```python
from build123d import *

# Parameters (mm, degrees)
F0_W     = 27
F0_H     = 31
F1_DEPTH = 2.5
F2_W     = 20.5
F2_H     = 31
F3_DEPTH = 2.5
F4_W     = 20.5
F4_H     = 31
F5_DEPTH = 2.5
F6_R     = 1.5
F7_DEPTH = 20.501
F8_R     = 1.5
F9_DEPTH = 32.001


with BuildPart() as f1:
    # F0 (on Right) → F1 (new body)
    with BuildSketch(Plane.YZ):
        Rectangle(F0_W, F0_H)
    extrude(amount=F1_DEPTH)

    # F2 (on face) → F3 (join)
    with BuildSketch(Plane(origin=(0, 13.5, 0), x_dir=(-1, 0, 0), z_dir=(0, 1, 0))):
        with Locations((7.75, 0)):
            Rectangle(F2_W, F2_H)
    extrude(amount=F3_DEPTH)

    # F4 (on face) → F5 (join)
    with BuildSketch(Plane.XZ.offset(13.5)):
        with Locations((-7.75, 0)):
            Rectangle(F4_W, F4_H)
    extrude(amount=F5_DEPTH)

    # F6 (on face) → F7 (cut, through all)
    with BuildSketch(Plane.YZ.offset(2.5)):
        with Locations((-10, -12)):
            Circle(F6_R)
        with Locations((-10, 12)):
            Circle(F6_R)
        with Locations((10, -12)):
            Circle(F6_R)
    extrude(amount=-F7_DEPTH, mode=Mode.SUBTRACT)

    # F8 (on face) → F9 (cut, through all)
    with BuildSketch(Plane.XZ.offset(16)):
        with Locations((-9, 10)):
            Circle(F8_R)
        with Locations((-9, -10)):
            Circle(F8_R)
    extrude(amount=-F9_DEPTH, mode=Mode.SUBTRACT)


solid = f1.part
```
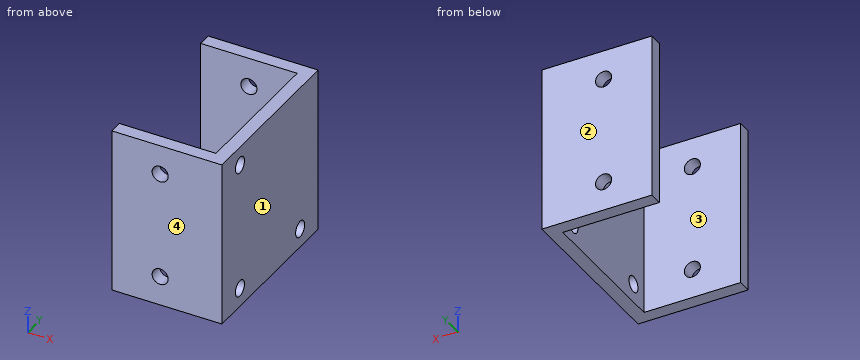
Verification items for the finished model (mm, model axes). Face numbers are marked on the shaded views. Coordinates: 2 decimals unless noted, no trailing zeros. Loops run counter-clockwise (first coordinate to the right, second up) from the corner with the lowest first, then second, coordinate; pieces in that order, holes last. Notation, with made-up numbers: (74, -39.75) - (101, -39.75) arc R22 cw to (101, -5.75) - close; hole circle Ø7 at (6.25, -1). An arc over 180 degrees is marked (long way). Return JSON: item names as keys, results as strings.
1. Section check D-D, the plane y = 10. Record the boundary of the cut face in (x, z).
Established:
{"outline": "(0, -15.5) - (2.5, -15.5) - (2.5, -13.5) - (0, -13.5) - close; (0, -10.5) - (2.5, -10.5) - (2.5, 15.5) - (0, 15.5) - close"}
2. Section check C-C, the plane z = -10. Record the boundary of the cut face in (x, y), then the cut area to 3 significant figures.
Established:
{"outline": "(-18, -16) - (-10.5, -16) - (-10.5, -13.5) - (-18, -13.5) - close; (-18, 13.5) - (-10.5, 13.5) - (-10.5, 16) - (-18, 16) - close; (-7.5, -16) - (2.5, -16) - (2.5, 16) - (-7.5, 16) - (-7.5, 13.5) - (0, 13.5) - (0, -13.5) - (-7.5, -13.5) - close", "area": "155 mm2"}
3. Go/stop test with flat-tipped pins: pin 1 (3.5 mm diameter, centred on y = 10, z = -12, fed in from +X); pin 2 (1 mm diameter, centred on y = -8.5, z = 7.5, fed in from -X). Record where each tip stops, or that it passes through.
Established:
{"pin 1": "stops at x = 2.5", "pin 2": "stops at x = 0"}
4. Section check A-A, the plane x = -9. Record the boundary of the cut face in (y, z), then the cut area to 3 significant figures.
Established:
{"outline": "(-16, -15.5) - (-13.5, -15.5) - (-13.5, -11.5) - (-16, -11.5) - close; (-16, -8.5) - (-13.5, -8.5) - (-13.5, 8.5) - (-16, 8.5) - close; (-16, 11.5) - (-13.5, 11.5) - (-13.5, 15.5) - (-16, 15.5) - close; (13.5, -15.5) - (16, -15.5) - (16, -11.5) - (13.5, -11.5) - close; (13.5, -8.5) - (16, -8.5) - (16, 8.5) - (13.5, 8.5) - close; (13.5, 11.5) - (16, 11.5) - (16, 15.5) - (13.5, 15.5) - close", "area": "125 mm2"}
5. Mould release check, pull along Y, two halves, no side actions. Record for the marked faces 1, 2, 3 and 4: +Y half, -Y half, draft (parallel to the pull), parting line (faces both ways), or undercut.
Established:
{"face 1": "draft", "face 2": "+Y half", "face 3": "undercut", "face 4": "-Y half"}
6. Section check B-B, the plane z = 12. Record the boundary of the cut face in (x, y).
Established:
{"outline": "(-18, -16) - (2.5, -16) - (2.5, -11.5) - (0, -11.5) - (0, -13.5) - (-18, -13.5) - close; (-18, 13.5) - (0, 13.5) - (0, -8.5) - (2.5, -8.5) - (2.5, 16) - (-18, 16) - close"}
7. Thickness scan on L1, parallel to Z at x = -9, y = -15.2; L2, parallel to Y at x = -8, z = 7; L3, parallel to Z at x = 1.1, y = -10. Record the ranges inside material, lowest first.
Established:
{"L1": "z = -15.5 to -11.5, -8.5 to 8.5, 11.5 to 15.5", "L2": "y = -16 to -13.5, 13.5 to 16", "L3": "z = -15.5 to -13.5, -10.5 to 10.5, 13.5 to 15.5"}
